```python
from build123d import *

# Parameters (mm, degrees)
SKETCH1_R           = 12.7
BOSS_EXTRUDE1_DEPTH = 8.89
SKETCH2_R           = 9.906
BOSS_EXTRUDE2_DEPTH = 69.85
FILLET2_R           = 1.27
CUT_EXTRUDE1_START  = -8.89
SKETCH5_W           = 28.368479266
SKETCH5_H           = 5.191734841
CUT_EXTRUDE1_DEPTH  = 69.85


with BuildPart() as part:
    # Sketch1 → Boss-Extrude1 (new body)
    with BuildSketch(Plane(origin=(0, 0, 0), x_dir=(1, 0, 0), z_dir=(0, 1, 0))):
        Circle(SKETCH1_R)
    extrude(amount=BOSS_EXTRUDE1_DEPTH)

    # Sketch2 → Boss-Extrude2 (add)
    with BuildSketch(Plane.XZ):
        Circle(SKETCH2_R)
    extrude(amount=BOSS_EXTRUDE2_DEPTH)

    # Fillet2
    fillet2_edges = [part.edges().sort_by_distance(p)[0] for p in [
        (-12.7, 8.89, 0),
    ]]
    fillet(fillet2_edges, radius=FILLET2_R)

    # Sketch5 → Cut-Extrude1 (cut)
    with BuildSketch(Plane.XY.offset(2.54).offset(CUT_EXTRUDE1_START)):
        with Locations((1.524929724, -63.573523151)):
            Rectangle(SKETCH5_W, SKETCH5_H)
    extrude(amount=-CUT_EXTRUDE1_DEPTH, mode=Mode.SUBTRACT)


solid = part.part
```
Source: CAD feature listing. Evaluate the final solid. Frame: model axes, mm. A direction names the side the tool comes from. Give positions to 0.01 mm unless a question says otherwise; leave off trailing zeros. Loops run counter-clockwise (first coordinate to the right, second up) from the corner with the lowest first, then second, coordinate; pieces in that order, holes last. Notation, with made-up numbers: (10, -12) -> (25, -12) arc R30 ccw to (25, 24) -> close; hole circle Ø2 at (21.5, 67.5). An arc over 180 degrees is marked (long way). Put each result on its own line as item: value. Start each with the question number.
1) Cut plane B-B (x = 0). Return loops of the section in (y, z).
2) Contact query for flat-ended pins moving along their axis: P1, Ø10, axis at x = -7, y = -34.5, coming from the -Z side; P2, Ø2.5, axis at x = -4, y = -63, coming from the -Z side; P3, Ø1.5, axis at x = -6.5, y = -8.5, coming from the +Z side. Output: stop coordinate, or through.
3) Cut plane A-A (z = 0). Return loops of the section in (x, y).
4) Material intervals for probe 1 along Y at (x, z) = (-8, -8); probe 2 along X at (y, z) = (-44, -3); probe 3 along Z at (x, y) = (-2, -34.5), sorted ascending.
5) Cut plane C-C (y = -62). Return loops of the section in (x, z).
6) Cut plane D-D (y = -42.5). Return loops of the section in (x, z).
7) Draft query along Y for faces 1 (the face through (0, -69.85, 0)), 2 (the face through (0, -64, -6.35)), 3 (the face through (0, 8.89, 0)). Return one class per face: released by +Y, released by -Y, zero draft, split by the parting line, or undercut.
8) Reachability of faces 4 (the face through (-8, 0, 7)), 5 (the face through (0, -66.169, -8)), 6 (the face through (-2.75, 3.76, 12.4)) from +Z, -Z, +X, -X, +Y, -Y: full face, straight path, thin tool, end or side. Return the list, or none.
Results are:
1. outline: (-69.85, -9.91) -> (-66.17, -9.91) -> (-66.17, -6.35) -> (-60.98, -6.35) -> (-60.98, -9.91) -> (0, -9.91) -> (0, -12.7) -> (7.62, -12.7) arc R1.27 ccw to (8.89, -11.43) -> (8.89, 11.43) arc R1.27 ccw to (7.62, 12.7) -> (0, 12.7) -> (0, 9.91) -> (-69.85, 9.91) -> close
2. P1: stops at z = -9.7
2. P2: stops at z = -6.35
2. P3: stops at z = 8.07
3. outline: (-12.7, 0) -> (-9.91, 0) -> (-9.91, -69.85) -> (9.91, -69.85) -> (9.91, 0) -> (12.7, 0) -> (12.7, 7.62) arc R1.27 ccw to (11.43, 8.89) -> (-11.43, 8.89) arc R1.27 ccw to (-12.7, 7.62) -> close
4. probe 1: y = 0 to 8.89
4. probe 2: x = -9.44 to 9.44
4. probe 3: z = -9.7 to 9.7
5. outline: (-7.6, -6.35) -> (7.6, -6.35) arc R9.91 ccw (long way) to start
6. outline: circle Ø19.81 at (0, 0)
7. face 1: released by -Y
7. face 2: undercut
7. face 3: released by +Y
8. face 4: -Y
8. face 5: -Z, +X, -X
8. face 6: +Y, -Y
